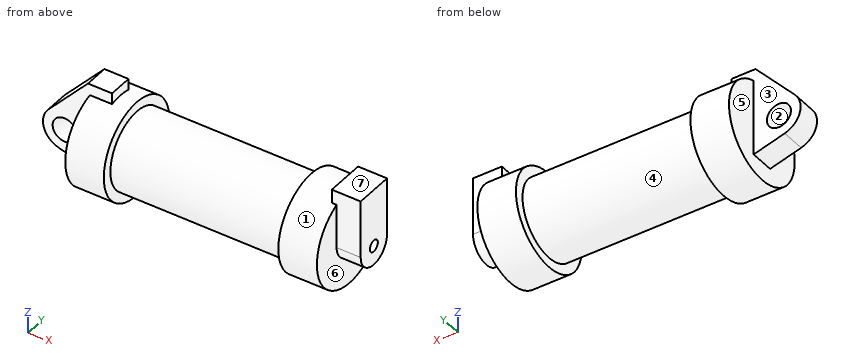
```python
from build123d import *

# Parameters (mm, degrees)
F0_W          = 5.842
F0_H          = 12.7
F2_R          = 1.524
F3_DEPTH      = 6.35
F3_DEPTH_BACK = 1.27
F4_DEPTH      = 56.134
F0_R          = 3.175
F5_DEPTH      = 3.175
F5_DEPTH_BACK = 3.175


with BuildPart() as f1:
    # F0 (on Front) → F1 (revolve)
    with BuildSketch(Plane.XZ):
        Polygon((5.842, 12.7), (5.842, 0), (66.294, 0), (66.294, 12.7), (56.134, 12.7), (56.134, 10.16), (10.16, 10.16), (10.16, 12.7), align=None)
        with Locations((2.921, 6.35)):
            Rectangle(F0_W, F0_H)
    revolve(axis=Axis((33.147, 0, 0), (-1, 0, 0)))

    # F2 (on face) → F3 (join, two sides)
    with BuildSketch(Plane.YZ.offset(66.294)) as f3_sk:
        with BuildLine():
            ThreePointArc((-5.08, 0), (0, -5.08), (5.08, 0))
            ThreePointArc((5.08, 0), (0, 5.08), (-5.08, 0))
        make_face()
        Circle(F2_R, mode=Mode.SUBTRACT)
        with BuildLine():
            ThreePointArc((-5.08, 0), (0, 5.08), (5.08, 0))
            Line((5.08, 0), (5.08, 15.24))
            Line((5.08, 15.24), (-5.08, 15.24))
            Line((-5.08, 15.24), (-5.08, 0))
        make_face()
    extrude(amount=F3_DEPTH)
    extrude(f3_sk.sketch, amount=-F3_DEPTH_BACK)

    # F2 (on face) → F4 (cut, through all)
    with BuildSketch(Plane.YZ.offset(66.294)):
        Circle(F2_R)
    extrude(amount=-F4_DEPTH, mode=Mode.SUBTRACT)

    # F0 (on Front) → F5 (join, two sides)
    with BuildSketch(Plane.XZ) as f5_sk:
        with BuildLine():
            Line((-0.9398, 0), (0, 0))
            Line((0, 0), (0, 12.7))
            Line((0, 12.7), (5.842, 12.7))
            Line((5.842, 12.7), (5.842, 15.24))
            Line((5.842, 15.24), (-0.508, 15.24))
            Line((-0.508, 15.24), (-10.88063, 3.847543))
            ThreePointArc((-10.88063, 3.847543), (-4.591961, 5.329721), (-0.9398, 0))
        make_face()
        with BuildLine():
            ThreePointArc((-8.182663, -5.506983), (-3.195791, -4.549339), (-0.9398, 0))
            ThreePointArc((-0.9398, 0), (-4.591961, 5.329721), (-10.88063, 3.847543))
            ThreePointArc((-10.88063, 3.847543), (-12.145978, -1.583727), (-8.182663, -5.506983))
        make_face()
        with Locations((-6.6548, 0)):
            Circle(F0_R, mode=Mode.SUBTRACT)
        with BuildLine():
            Line((5.842, 0), (0, 0))
            Line((0, 0), (-0.9398, 0))
            ThreePointArc((-0.9398, 0), (-3.195791, -4.549339), (-8.182663, -5.506983))
            Line((-8.182663, -5.506983), (5.842, -9.398))
            Line((5.842, -9.398), (5.842, 0))
        make_face()
        with Locations((2.921, 6.35)):
            Rectangle(F0_W, F0_H)
    extrude(amount=F5_DEPTH)
    extrude(f5_sk.sketch, amount=-F5_DEPTH_BACK)


solid = f1.part
```
The model under review builds one solid part; all positions refer to its coordinate system, in mm. Face numbers are marked on the shaded views. A direction names the side the tool comes from. Coordinates: 2 decimals unless noted, no trailing zeros. Write each loop counter-clockwise with the first axis right and the second up, starting at its lowest first coordinate (ties: lowest second). Pieces come first, ordered by that corner, then holes.
1) To check wall thickness, follow probe 1 along X at (y, z) = (2.25, 10); probe 2 along Z at (x, y) = (60, 0); probe 3 along Y at (x, z) = (55.5, 0.75). State the ranges of each line that lie inside material, in increasing order.
2) We need section D-D on x = 2. State the section outline as (y, z) points (3 decimals), then the cut area to 3 significant figures.
3) Clearance check with flat-ended pins moving along their axes: pin 1 Ø12 at (x, z) = (21, -2.5) entering from -Y; pin 2 Ø2.5 at (x, z) = (67, 11) entering from +Y; pin 3 Ø12 at (x, y) = (54, 8) entering from +Z; pin 4 Ø1.5 at (x, z) = (24.5, 11.5) entering from -Y. State where each tip first meets the part, or that it passes through.
4) We need section C-C on x = 51.5. State the section outline as (y, z) points, then the cut area to 3 significant figures.
5) The part is to be moulded in two halves that separate along Z. For the marked faces 1, 2 and 3, say which applies: pulls with the +Z half, pulls with the -Z half, needs draft (parallel to the pull), parting line crosses it, or undercut.
6) We need section B-B on y = 6.5. State the section outline as (x, z) points.
7) We need section A-A on y = 0. State the section outline as (x, z) points (3 decimals), then the cut area to 3 significant figures.
8) Machinability: for the marked faces 4, 5, 6 and 7, which of the approach directions +Z, -Z, +X, -X, +Y, -Y give a long, thin tool a straight path to every point of the face, cutting with its end or side? Answer none if there is none.
Answer list:
1. probe 1: x = -5.28 to 10.16, 56.13 to 72.64
1. probe 2: z = -12.7 to -1.52, 1.52 to 12.7
1. probe 3: y = -10.13 to -1.33, 1.33 to 10.13
2. outline: (-3.175, 12.297) arc R12.7 ccw (long way) to (3.175, 12.297) - (3.175, 15.24) - (-3.175, 15.24) - close
2. area: 524 mm2
3. pin 1: stops at y = -10.16
3. pin 2: stops at y = 7.87
3. pin 3: stops at z = 12.47
3. pin 4: passes through
4. outline: circle Ø20.32 at (0, 0); hole circle Ø3.05 at (0, 0)
4. area: 317 mm2
5. face 1: parting line crosses it
5. face 2: undercut
5. face 3: needs draft
6. outline: (0, -10.91) - (10.16, -10.91) - (10.16, -7.81) - (56.13, -7.81) - (56.13, -10.91) - (66.29, -10.91) - (66.29, 10.91) - (56.13, 10.91) - (56.13, 7.81) - (10.16, 7.81) - (10.16, 10.91) - (0, 10.91) - close
7. outline: (-10.881, 3.848) arc R5.715 ccw to (-8.183, -5.507) - (0, -7.777) - (0, -12.7) - (10.16, -12.7) - (10.16, -10.16) - (56.134, -10.16) - (56.134, -12.7) - (66.294, -12.7) - (66.294, -5.08) - (72.644, -5.08) - (72.644, -1.524) - (10.16, -1.524) - (10.16, 1.524) - (72.644, 1.524) - (72.644, 15.24) - (65.024, 15.24) - (65.024, 12.7) - (56.134, 12.7) - (56.134, 10.16) - (10.16, 10.16) - (10.16, 12.7) - (5.842, 12.7) - (5.842, 15.24) - (-0.508, 15.24) - close; hole circle Ø6.35 at (-6.655, 0)
7. area: 1,560 mm2
8. face 4: none
8. face 5: -Z, -X
8. face 6: -Z, +X
8. face 7: +Z, +X, -X, +Y, -Y
